from build123d import *

# Parameters (mm, degrees)
MAIN_EXTRUSION_DEPTH      = 1.6
MAIN_EXTRUSION_DEPTH_BACK = 3
TAPERED_BOTTOM_DEPTH      = 2
TAPERED_BOTTOM_TAPER      = 45
PCB_SUPPORT_REACH         = 7
SKETCH4_R                 = 2.795
SKETCH4_W                 = 2.75
SKETCH4_H                 = 22.09
SKETCH4_W_2               = 8
SKETCH4_H_2               = 5.25
SKETCH5_R                 = 1.545
GUIDE_PINS_DEPTH          = 3
GUIDE_PINS_TAPER          = 7.5


with BuildPart() as part:
    # Sketch2 → main-extrusion (new body, two sides)
    with BuildSketch(Plane(origin=(0, 0, 0), x_dir=(1, 0, 0), z_dir=(0, 1, 0))) as main_extrusion_sk:
        with BuildLine():
            Line((-2.25, 19.36), (-2.25, 2.23))
            ThreePointArc((-2.25, 2.23), (-0.93783838, -0.93783838), (2.23, -2.25))
            Line((2.23, -2.25), (29.52, -2.25))
            ThreePointArc((29.52, -2.25), (32.68783838, -0.93783838), (34, 2.23))
            Line((34, 2.23), (34, 19.36))
            ThreePointArc((34, 19.36), (32.68783838, 22.52783838), (29.52, 23.84))
            Line((29.52, 23.84), (2.23, 23.84))
            ThreePointArc((2.23, 23.84), (-0.93783838, 22.52783838), (-2.25, 19.36))
        make_face()
        with BuildLine():
            Line((-0.25, 19.36), (-0.25, 2.23))
            ThreePointArc((-0.25, 2.23), (0.476375183, 0.476375183), (2.23, -0.25))
            Line((2.23, -0.25), (29.52, -0.25))
            ThreePointArc((29.52, -0.25), (31.273624817, 0.476375183), (32, 2.23))
            Line((32, 2.23), (32, 19.36))
            ThreePointArc((32, 19.36), (31.273624817, 21.113624817), (29.52, 21.84))
            Line((29.52, 21.84), (2.23, 21.84))
            ThreePointArc((2.23, 21.84), (0.476375183, 21.113624817), (-0.25, 19.36))
        make_face(mode=Mode.SUBTRACT)
    extrude(amount=MAIN_EXTRUSION_DEPTH)
    extrude(main_extrusion_sk.sketch, amount=-MAIN_EXTRUSION_DEPTH_BACK)

    # Sketch3 → tapered-bottom (add)
    with BuildSketch(Plane.XZ.offset(3)):
        with BuildLine():
            ThreePointArc((-2.25, -19.36), (-0.93783838, -22.52783838), (2.23, -23.84))
            Line((2.23, -23.84), (29.52, -23.84))
            ThreePointArc((29.52, -23.84), (32.68783838, -22.52783838), (34, -19.36))
            Line((34, -19.36), (34, -2.23))
            ThreePointArc((34, -2.23), (32.68783838, 0.93783838), (29.52, 2.25))
            Line((29.52, 2.25), (2.23, 2.25))
            ThreePointArc((2.23, 2.25), (-0.93783838, 0.93783838), (-2.25, -2.23))
            Line((-2.25, -2.23), (-2.25, -19.36))
        make_face()
    extrude(amount=TAPERED_BOTTOM_DEPTH, taper=TAPERED_BOTTOM_TAPER)

    # Sketch4 → PCB-support (add, up to next)
    with BuildSketch(Plane(origin=(0, 0, 0), x_dir=(1, 0, 0), z_dir=(0, 1, 0)), mode=Mode.PRIVATE) as pcb_support_sk1:
        with Locations((27.94, 19.05)):
            Circle(SKETCH4_R)
    pcb_support_tool1 = extrude(pcb_support_sk1.sketch, amount=-PCB_SUPPORT_REACH, mode=Mode.PRIVATE) - part.part
    add(pcb_support_tool1.solids().sort_by_distance((27.94, 0, -19.05))[0])
    # Sketch4 → PCB-support (add, up to next)
    with BuildSketch(Plane(origin=(0, 0, 0), x_dir=(1, 0, 0), z_dir=(0, 1, 0)), mode=Mode.PRIVATE) as pcb_support_sk2:
        with Locations((27.94, 2.54)):
            Circle(SKETCH4_R)
    pcb_support_tool2 = extrude(pcb_support_sk2.sketch, amount=-PCB_SUPPORT_REACH, mode=Mode.PRIVATE) - part.part
    add(pcb_support_tool2.solids().sort_by_distance((27.94, 0, -2.54))[0])
    # Sketch4 → PCB-support (add, up to next)
    with BuildSketch(Plane(origin=(0, 0, 0), x_dir=(1, 0, 0), z_dir=(0, 1, 0)), mode=Mode.PRIVATE) as pcb_support_sk3:
        with Locations((1.125, 10.795)):
            Rectangle(SKETCH4_W, SKETCH4_H)
    pcb_support_tool3 = extrude(pcb_support_sk3.sketch, amount=-PCB_SUPPORT_REACH, mode=Mode.PRIVATE) - part.part
    add(pcb_support_tool3.solids().sort_by_distance((1.125, 0, -10.795))[0])
    # Sketch4 → PCB-support (add, up to next)
    with BuildSketch(Plane(origin=(0, 0, 0), x_dir=(1, 0, 0), z_dir=(0, 1, 0)), mode=Mode.PRIVATE) as pcb_support_sk4:
        with Locations((13, 19.215)):
            Rectangle(SKETCH4_W_2, SKETCH4_H_2)
    pcb_support_tool4 = extrude(pcb_support_sk4.sketch, amount=-PCB_SUPPORT_REACH, mode=Mode.PRIVATE) - part.part
    add(pcb_support_tool4.solids().sort_by_distance((13, 0, -19.215))[0])
    # Sketch4 → PCB-support (add, up to next)
    with BuildSketch(Plane(origin=(0, 0, 0), x_dir=(1, 0, 0), z_dir=(0, 1, 0)), mode=Mode.PRIVATE) as pcb_support_sk5:
        with Locations((13, 2.375)):
            Rectangle(SKETCH4_W_2, SKETCH4_H_2)
    pcb_support_tool5 = extrude(pcb_support_sk5.sketch, amount=-PCB_SUPPORT_REACH, mode=Mode.PRIVATE) - part.part
    add(pcb_support_tool5.solids().sort_by_distance((13, 0, -2.375))[0])

    # Sketch5 → guide-pins (add)
    with BuildSketch(Plane(origin=(0, 0, 0), x_dir=(1, 0, 0), z_dir=(0, 1, 0))):
        with Locations((27.94, 19.05)):
            Circle(SKETCH5_R)
        with Locations((27.94, 2.54)):
            Circle(SKETCH5_R)
    extrude(amount=GUIDE_PINS_DEPTH, taper=GUIDE_PINS_TAPER)

    # top-ridge: sweep along a path in path
    with BuildLine(Plane(origin=(0, 1.6, 0), x_dir=(1, 0, 0), z_dir=(0, 1, 0))) as top_ridge_path:
        Line((2.23, -0.25), (29.52, -0.25))
        ThreePointArc((29.52, -0.25), (31.273624817, 0.476375183), (32, 2.23))
        Line((32, 2.23), (32, 19.36))
        ThreePointArc((32, 19.36), (31.273624817, 21.113624817), (29.52, 21.84))
        Line((29.52, 21.84), (2.23, 21.84))
        ThreePointArc((2.23, 21.84), (0.476375183, 21.113624817), (-0.25, 19.36))
        Line((-0.25, 19.36), (-0.25, 2.23))
        ThreePointArc((-0.25, 2.23), (0.476375183, 0.476375183), (2.23, -0.25))
    # profile → top-ridge (sweep, cut)
    with BuildSketch(Plane(origin=(2.23, 0, 0), x_dir=(0, 0, -1), z_dir=(1, 0, 0))):
        with BuildLine():
            Line((-2.25, 1.6), (-2.25, -1.4))
            Line((-2.25, -1.4), (-1.25, -1.4))
            Line((-1.25, -1.4), (-1.25, 0.35))
            ThreePointArc((-1.25, 0.35), (-1.55, 0.85), (-1.25, 1.35))
            Line((-1.25, 1.35), (-1.25, 1.6))
            Line((-1.25, 1.6), (-2.25, 1.6))
        make_face()
    sweep(path=top_ridge_path.line, mode=Mode.SUBTRACT)


solid = part.part
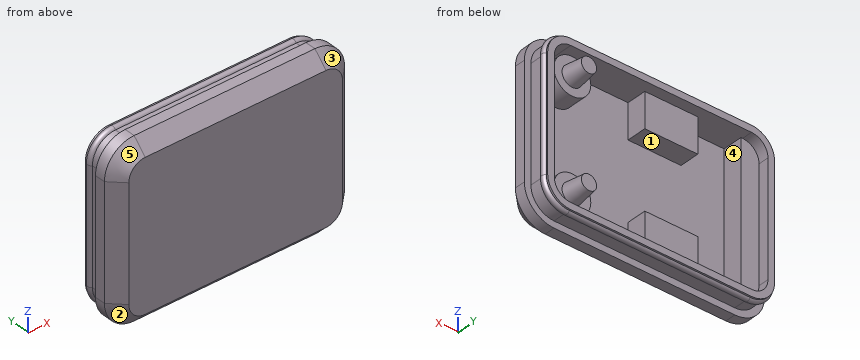
Source: CAD feature listing. Evaluate the final solid. Frame: model axes, mm. Face numbers are marked on the shaded views. A direction names the side the tool comes from. Give positions to 0.01 mm unless a question says otherwise; leave off trailing zeros. Write each loop counter-clockwise with the first axis right and the second up, starting at its lowest first coordinate (ties: lowest second). Pieces come first, ordered by that corner, then holes. Notation, with made-up numbers: (-37.75, 48) -> (-23.75, 48) arc R24 ccw to (-23.75, 77) -> close; hole circle Ø1 at (17, 85). An arc over 180 degrees is marked (long way). Return JSON: item names as keys, results as strings. Group by question number.
1. Material intervals for line 1 (Z direction, x = 15, y = -1.25); line 2 (Z direction, x = 20, y = 0.75); line 3 (X direction, y = -1.5, z = -8), sorted ascending. Write a range as from..to.
2. Pin query (flat end, axial travel): pin 1 Ø7 at (x, z) = (15.5, -8) entering from +Y; pin 2 Ø1.5 at (x, z) = (15, -15) entering from +Y; pin 3 Ø2 at (x, z) = (0.5, -11) entering from +Y. Return the tip coordinate at first contact, or that it passes through.
3. Mould query, pull axis X, two halves, no side actions, for the marked faces 3, 4 and 5. Classes: +X half, -X half, draft (parallel to the pull), parting line (faces both ways), or undercut.
4. Section A-A, the plane y = 2. Output: boundary loops of the cut face in (x, z).
5. Access query for the marked faces 1 and 2. Directions: +Z, -Z, +X, -X, +Y, -Y. A direction counts if a zero-diameter tool reaches every point of the face in a straight line with its end or side. Return the directions, or none.
Determined:
{
 "1": {"line 1": "z = -22.84..-16.59, -5..1.25", "line 2": "z = -23.13..-21.84, 0.25..1.54", "line 3": "x = -2.25..2.5, 32..34"},
 "2": {"pin 1": "stops at y = 0", "pin 2": "stops at y = -3", "pin 3": "stops at y = 1.6"},
 "3": {"face 3": "+X half", "face 4": "undercut", "face 5": "-X half"},
 "4": {"outline": "circle Ø2.56 at (27.94, -19.05); circle Ø2.56 at (27.94, -2.54)"},
 "5": {"face 1": "+Y", "face 2": "-Z, -X, -Y"}
}
